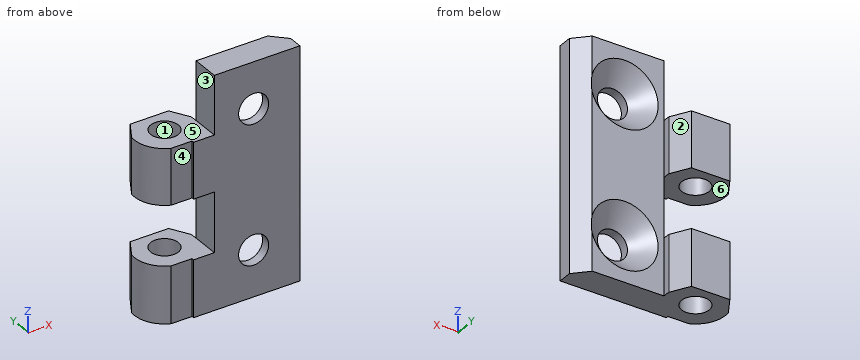
from build123d import *

# Parameters (mm, degrees)
SKETCH2_R           = 3
BOSS_EXTRUDE1_DEPTH = 25
SKETCH3_R           = 3.25
CUT_EXTRUDE1_DEPTH  = 36.860842154
CHAMFER1_SIZE       = 4
CUT_EXTRUDE2_DEPTH  = 57.278326201
SKETCH5_W           = 13
SKETCH5_H           = 12.5
CUT_EXTRUDE3_DEPTH  = 38.17862289
SKETCH6_W           = 13
SKETCH6_H           = 0.2
CUT_EXTRUDE4_DEPTH  = 38.17862289


with BuildPart() as part:
    # Sketch2 → Boss-Extrude1 (new, symmetric)
    with BuildSketch(Plane.XY):
        with BuildLine():
            Line((25, -6.5), (2, -6.5))
            Line((2, -6.5), (2, -6))
            Line((2, -6), (-2.5, -6))
            ThreePointArc((-2.5, -6), (-6.427802106, -0.966105629), (-4.153311931, 5))
            Line((-4.153311931, 5), (4.153311931, 5))
            ThreePointArc((4.153311931, 5), (5.986089611, 2.533126757), (6.480740698, -0.5))
            Line((6.480740698, -0.5), (22, -0.5))
            Line((22, -0.5), (25, -3.5))
            Line((25, -3.5), (25, -6.5))
        make_face()
        Circle(SKETCH2_R, mode=Mode.SUBTRACT)
    extrude(amount=BOSS_EXTRUDE1_DEPTH, both=True)

    # Sketch3 → Cut-Extrude1 (cut, through all)
    with BuildSketch(Plane(origin=(0, -0.5, 0), x_dir=(1, 0, 0), z_dir=(0, 1, 0))):
        with Locations(Location((15, 15, 0), (0, 0, 180))):
            Circle(SKETCH3_R)
        with Locations(Location((15, -15, 0), (0, 0, 180))):
            Circle(SKETCH3_R)
    extrude(amount=-CUT_EXTRUDE1_DEPTH, mode=Mode.SUBTRACT)

    # Chamfer1
    # the kernel refuses this chamfer: 4 mm, written as the material it takes off along each edge
    with BuildSketch(Plane(origin=(15, -0.5, -15), x_dir=(-1, 0, 0), z_dir=(0, 0, -1))) as chamfer1_piece_1:
        Polygon((3.25, -CHAMFER1_SIZE), (3.25 + CHAMFER1_SIZE, 0), (3.25, 0), align=None)
    revolve(axis=Axis((15, -0.5, -15), (0, 1, 0)), mode=Mode.SUBTRACT)
    with BuildSketch(Plane(origin=(15, -0.5, 15), x_dir=(-1, 0, 0), z_dir=(0, 0, -1))) as chamfer1_piece_2:
        Polygon((3.25, -CHAMFER1_SIZE), (3.25 + CHAMFER1_SIZE, 0), (3.25, 0), align=None)
    revolve(axis=Axis((15, -0.5, 15), (0, 1, 0)), mode=Mode.SUBTRACT)

    # Sketch4 → Cut-Extrude2 (cut, through all)
    with BuildSketch(Plane.XY.offset(25)):
        with BuildLine():
            Line((6.406782985, 1.096873642), (4.153311931, 5))
            ThreePointArc((4.153311931, 5), (5.629165125, 3.25), (6.406782985, 1.096873642))
        make_face()
        with BuildLine():
            Line((-4.153311931, 5), (-6.406782985, 1.096873642))
            ThreePointArc((-6.406782985, 1.096873642), (-5.629165125, 3.25), (-4.153311931, 5))
        make_face()
    extrude(amount=-CUT_EXTRUDE2_DEPTH, mode=Mode.SUBTRACT)

    # Sketch5 → Cut-Extrude3 (cut, through all)
    with BuildSketch(Plane(origin=(0, 5, 0), x_dir=(1, 0, 0), z_dir=(0, 1, 0))):
        with Locations((0, -18.75)):
            Rectangle(SKETCH5_W, SKETCH5_H)
        with Locations((0, 6.25)):
            Rectangle(SKETCH5_W, SKETCH5_H)
    extrude(amount=-CUT_EXTRUDE3_DEPTH, mode=Mode.SUBTRACT)

    # Sketch6 → Cut-Extrude4 (cut, through all)
    with BuildSketch(Plane(origin=(0, 5, 0), x_dir=(1, 0, 0), z_dir=(0, 1, 0))):
        with Locations((0, -0.1)):
            Rectangle(SKETCH6_W, SKETCH6_H)
        with Locations((0, -12.4)):
            Rectangle(SKETCH6_W, SKETCH6_H)
        with Locations((0, 12.6)):
            Rectangle(SKETCH6_W, SKETCH6_H)
    extrude(amount=-CUT_EXTRUDE4_DEPTH, mode=Mode.SUBTRACT)


solid = part.part
CAD build for the part. Positions are in the model's coordinates, mm. Face numbers are marked on the shaded views. A direction names the side the tool comes from. Coordinates: 2 decimals unless noted, no trailing zeros. Order: outer loops, then holes, each group sorted by start corner. A loop starts at its lowest first (then second) coordinate and runs counter-clockwise, first axis right, second up. Notation, with made-up numbers: (1, 11) -> (48, 11) arc R15 ccw to (48, 26) -> close; hole circle Ø8 at (79.5, 5.25). An arc over 180 degrees is marked (long way). Answer in a Markdown table with one row per item.
1) Drill centre lines: line 1 (Z direction, x = 15, y = -4.9); line 2 (X direction, y = 0, z = 4.5); line 3 (Z direction, x = 16, y = -4.5). Where is each one in solid material? Low to high.
Check values:
| item | result |
|---|---|
| line 1 | -25 to -18.25, -11.75 to 11.75, 18.25 to 25 |
| line 2 | -6.5 to -3, 3 to 6.5 |
| line 3 | -25 to -18.09, -11.91 to 11.91, 18.09 to 25 |
2) Band-saw the part on D-D (x = 15). List the corners of the cut face in (y, z), and give its area (3 significant figures).
Check values:
| item | result |
|---|---|
| outline | (-6.5, -25) -> (-0.5, -25) -> (-0.5, -22.25) -> (-4.5, -18.25) -> (-6.5, -18.25) -> close; (-6.5, -11.75) -> (-4.5, -11.75) -> (-0.5, -7.75) -> (-0.5, 7.75) -> (-4.5, 11.75) -> (-6.5, 11.75) -> close; (-6.5, 18.25) -> (-4.5, 18.25) -> (-0.5, 22.25) -> (-0.5, 25) -> (-6.5, 25) -> close |
| area | 190 mm2 |
3) Which spindle directions (+Z, -Z, +X, -X, +Y, -Y) get a long thin tool onto all of the face, cutting with end or side? Do the marked faces 4, 5 and 6. Say none if no direction does.
Check values:
| item | result |
|---|---|
| face 4 | +Z, -Z, -X, -Y |
| face 5 | +Z, -X, +Y, -Y |
| face 6 | -X, +Y, -Y |
4) Band-saw the part on C-C (y = -2.25). List the corners of the cut face in (x, z).
Check values:
| item | result |
|---|---|
| outline | (-6.1, -25) -> (-1.98, -25) -> (-1.98, -12.7) -> (-6.1, -12.7) -> close; (-6.1, 0.2) -> (-1.98, 0.2) -> (-1.98, 12.3) -> (-6.1, 12.3) -> close; (1.98, -25) -> (23.75, -25) -> (23.75, 25) -> (6.5, 25) -> (6.5, 12.3) -> (1.98, 12.3) -> (1.98, 0.2) -> (6.5, 0.2) -> (6.5, -12.7) -> (1.98, -12.7) -> close; hole circle Ø11 at (15, -15); hole circle Ø11 at (15, 15) |
5) Band-saw the part on A-A (x = 0). List the corners of the cut face in (y, z).
Check values:
| item | result |
|---|---|
| outline | (-6, -25) -> (-3, -25) -> (-3, -12.7) -> (-6, -12.7) -> close; (-6, 0.2) -> (-3, 0.2) -> (-3, 12.3) -> (-6, 12.3) -> close; (3, -25) -> (5, -25) -> (5, -12.7) -> (3, -12.7) -> close; (3, 0.2) -> (5, 0.2) -> (5, 12.3) -> (3, 12.3) -> close |
6) Band-saw the part on B-B (z = 6.5). List the corners of the cut face in (x, y).
Check values:
| item | result |
|---|---|
| outline | (-6.41, 1.1) arc R6.5 ccw to (-2.5, -6) -> (2, -6) -> (2, -6.5) -> (25, -6.5) -> (25, -3.5) -> (22, -0.5) -> (6.48, -0.5) arc R6.5 ccw to (6.41, 1.1) -> (4.15, 5) -> (-4.15, 5) -> close; hole circle Ø6 at (0, 0) |
7) Mould opens along Y. For the marked faces 1, 2 and 3 say: pulls with the +Y half, pulls with the -Y half, needs draft (parallel to the pull), parting line crosses it, or undercut.
Check values:
| item | result |
|---|---|
| face 1 | undercut |
| face 2 | pulls with the +Y half |
| face 3 | needs draft |
8) Flat gauge pins, fed straight in: P1, Ø10, axis at x = 13, z = 2, coming from the +Y side; P2, Ø5, axis at x = 15, z = 15, coming from the -Y side; P3, Ø3.5, axis at x = -2.5, y = -2, coming from the +Z side; P4, Ø4, axis at y = 0.5, z = -4, coming from the -X side. Where does each tip first touch, or does it go through?
Check values:
| item | result |
|---|---|
| P1 | y = -0.5 |
| P2 | through |
| P3 | z = 12.3 |
| P4 | x = 6.5 |
